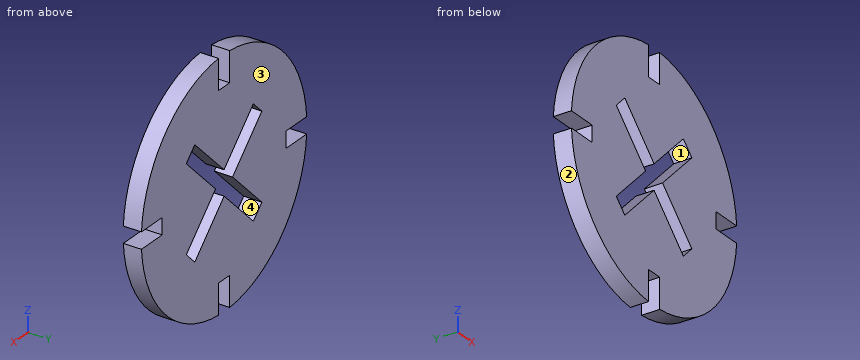
from build123d import *

# Parameters (mm, degrees)
BOSS_EXTRUDE1_DEPTH = 3
CUT_EXTRUDE1_REACH  = 5


with BuildPart() as part:
    # Sketch1 → Boss-Extrude1 (new body)
    with BuildSketch(Plane(origin=(0, 0, 0), x_dir=(1, 0, 0), z_dir=(0, 1, 0))):
        with BuildLine():
            Line((1.35, 14.954385483), (-1.35, 14.954385483))
            Line((-1.35, 14.954385483), (-1.35, 19.954385483))
            ThreePointArc((-1.35, 19.954385483), (-14.142135624, 14.142135624), (-19.954385483, 1.35))
            Line((-19.954385483, 1.35), (-14.954385483, 1.35))
            Line((-14.954385483, 1.35), (-14.954385483, -1.35))
            Line((-14.954385483, -1.35), (-19.954385483, -1.35))
            ThreePointArc((-19.954385483, -1.35), (-14.142135624, -14.142135624), (-1.35, -19.954385483))
            Line((-1.35, -19.954385483), (-1.35, -14.954385483))
            Line((-1.35, -14.954385483), (1.35, -14.954385483))
            Line((1.35, -14.954385483), (1.35, -19.954385483))
            ThreePointArc((1.35, -19.954385483), (14.142135624, -14.142135624), (19.954385483, -1.35))
            Line((19.954385483, -1.35), (14.954385483, -1.35))
            Line((14.954385483, -1.35), (14.954385483, 1.35))
            Line((14.954385483, 1.35), (19.954385483, 1.35))
            ThreePointArc((19.954385483, 1.35), (14.142135624, 14.142135624), (1.35, 19.954385483))
            Line((1.35, 19.954385483), (1.35, 14.954385483))
        make_face()
    extrude(amount=BOSS_EXTRUDE1_DEPTH)

    # Sketch3 → Cut-Extrude1 (cut, up to next)
    with BuildSketch(Plane(origin=(0, 3, 0), x_dir=(1, 0, 0), z_dir=(0, 1, 0)), mode=Mode.PRIVATE) as cut_extrude1_sk1:
        Polygon((0, 2.050609665), (7.071067812, 9.121677477), (9.121677477, 7.071067812), (2.050609665, 0), (9.121677477, -7.071067812), (7.071067812, -9.121677477), (0, -2.050609665), (-7.071067812, -9.121677477), (-9.121677477, -7.071067812), (-2.050609665, 0), (-9.121677477, 7.071067812), (-7.071067812, 9.121677477), align=None)
    cut_extrude1_tool1 = extrude(cut_extrude1_sk1.sketch, amount=-CUT_EXTRUDE1_REACH, mode=Mode.PRIVATE) & part.part
    add(cut_extrude1_tool1.solids().sort_by_distance((0, 3, 0))[0], mode=Mode.SUBTRACT)


solid = part.part
The listing builds one solid part. Answer for the finished solid, in the listing's coordinates (mm). Face numbers are marked on the shaded views. Round coordinates to 2 decimals unless told otherwise and drop trailing zeros. Write each loop counter-clockwise with the first axis right and the second up, starting at its lowest first coordinate (ties: lowest second). Pieces come first, ordered by that corner, then holes. Notation, with made-up numbers: M -8.5,81 L 41.5,81 A13 cw 41.5,104 Z; hole C 12,71 d1. An arc over 180 degrees is marked long. Write each question's results on one line, items separated by ' | '. Start each with the question number.
Item 1: Flat-ended cylindrical pins translate along their axes: pin 1 Ø1.5 at (x, y) = (-18.5, 1.5) entering from +Z; pin 2 Ø1.5 at (y, z) = (2, -16.5) entering from -X; pin 3 Ø1.4 at (y, z) = (2, 0) entering from +X. Find the tip coordinate at first contact, or state that the pin passes through.
Item 2: Straight lines are drawn through the part: L1, parallel to Z at x = -5, y = 1.75; L2, parallel to Z at x = 6.5, y = 0.25; L3, parallel to X at y = 0.15, z = 7 (3 decimals). For each, find the intervals that lie inside material, in ascending order. Write a range as [from, to].
Item 3: A cutting plane is placed at A-A on x = -16. Write down the section's boundary in (y, z), and give its area (3 significant figures).
Item 4: A cutting plane is placed at C-C on z = -4.5. Write down the section's boundary in (x, y).
Item 5: A cutting plane is placed at B-B on y = 2.45. Write down the section's boundary in (x, z), and give its area (3 significant figures).
Item 6: A cutting plane is placed at D-D on x = -3. Write down the section's boundary in (y, z), and give its area (3 significant figures).
Item 7: For a pull along X with two mould halves and no side action, classify the marked faces 1, 2, 3 and 4 as pulls with the +X half, pulls with the -X half, needs draft (parallel to the pull), parting line crosses it, or undercut.
Check sheet entries:
1) pin 1: z = 9.22 | pin 2: x = -12.33 | pin 3: x = 14.95
2) L1: [-19.36, -7.05], [-2.95, 2.95], [7.05, 19.36] | L2: [-18.91, -8.55], [-4.45, 4.45], [8.55, 18.91] | L3: [-18.735, -9.051], [-4.949, 4.949], [9.051, 18.735]
3) outline: M 0,-12 L 3,-12 L 3,-1.35 L 0,-1.35 Z; M 0,1.35 L 3,1.35 L 3,12 L 0,12 Z | area: 63.9 mm²
4) outline: M -19.49,0 L -6.55,0 L -6.55,3 L -19.49,3 Z; M -2.45,0 L 2.45,0 L 2.45,3 L -2.45,3 Z; M 6.55,0 L 19.49,0 L 19.49,3 L 6.55,3 Z
5) outline: M -19.95,-1.35 A20 ccw -1.35,-19.95 L -1.35,-14.95 L 1.35,-14.95 L 1.35,-19.95 A20 ccw 19.95,-1.35 L 14.95,-1.35 L 14.95,1.35 L 19.95,1.35 A20 ccw 1.35,19.95 L 1.35,14.95 L -1.35,14.95 L -1.35,19.95 A20 ccw -19.95,1.35 L -14.95,1.35 L -14.95,-1.35 Z; hole M -9.12,-7.07 L -7.07,-9.12 L 0,-2.05 L 7.07,-9.12 L 9.12,-7.07 L 2.05,0 L 9.12,7.07 L 7.07,9.12 L 0,2.05 L -7.07,9.12 L -9.12,7.07 L -2.05,0 Z | area: 1,080 mm²
6) outline: M 0,-19.77 L 3,-19.77 L 3,-5.05 L 0,-5.05 Z; M 0,-0.95 L 3,-0.95 L 3,0.95 L 0,0.95 Z; M 0,5.05 L 3,5.05 L 3,19.77 L 0,19.77 Z | area: 94.0 mm²
7) face 1: undercut | face 2: pulls with the -X half | face 3: needs draft | face 4: undercut
